Could you check a few things on this model? Use its own coordinates, in mm. Give positions to 0.01 mm unless a question says otherwise; leave off trailing zeros. Loops run counter-clockwise (first coordinate to the right, second up) from the corner with the lowest first, then second, coordinate; pieces in that order, holes last. Notation, with made-up numbers: M -30,67 L -12,67 A22 ccw -12,100 Z; hole C -17,34 d11. An arc over 180 degrees is marked long. Use a Markdown table: item, result. Add a question column.
1) Will this pin go through, and if not, where does the flat tip stop? pin 1 Ø3 at (x, y) = (0, 34.925) entering from +Z.
2) If I drill on line 1 along Y through (x, z) = (-11, 1.55) (3 decimals); line 2 along Y through (x, z) = (-8, 2.8) (3 decimals); line 3 along X through (y, z) = (30, 2.55), over which ranges is the centre line in solid material (lowest first)? Write a range as [from, to].
3) Suppose I cut it at A-A on y = 36. List the corners of the cut face in (x, z) for me (3 decimals), and give its area (3 significant figures).
```python
from build123d import *

# Parameters (mm, degrees)
F0_R     = 2.3749
F1_DEPTH = 3.175
F3_DEPTH = 25.4


with BuildPart() as f1:
    # F0 (on Top) → F1 (new body)
    with BuildSketch(Plane.XY):
        with BuildLine():
            Line((-38.1, -9.525), (38.1, -9.525))
            Line((38.1, -9.525), (38.1, 28.575))
            ThreePointArc((38.1, 28.575), (34.380256, 37.555256), (25.4, 41.275))
            Line((25.4, 41.275), (3.322108, 41.275))
            Line((3.322108, 41.275), (-25.4, 41.275))
            ThreePointArc((-25.4, 41.275), (-34.380256, 37.555256), (-38.1, 28.575))
            Line((-38.1, 28.575), (-38.1, -9.525))
        make_face()
        with Locations((0, 34.925)):
            Circle(F0_R, mode=Mode.SUBTRACT)
    extrude(amount=F1_DEPTH)

    # F2 (on face) → F3 (cut)
    with BuildSketch(Plane.XY.offset(3.175)):
        Polygon((-38.1, -7.62), (-38.1, -14.148636), (38.1, -14.148636), (38.1, -7.62), (37.1475, -9.525), (36.195, -7.62), (35.2425, -9.525), (34.29, -7.62), (33.3375, -9.525), (32.385, -7.62), (31.4325, -9.525), (30.48, -7.62), (29.5275, -9.525), (28.575, -7.62), (27.6225, -9.525), (26.67, -7.62), (25.7175, -9.525), (24.765, -7.62), (23.8125, -9.525), (22.86, -7.62), (21.9075, -9.525), (20.955, -7.62), (20.0025, -9.525), (19.05, -7.62), (18.0975, -9.525), (17.145, -7.62), (16.1925, -9.525), (15.24, -7.62), (14.2875, -9.525), (13.335, -7.62), (12.3825, -9.525), (11.43, -7.62), (10.4775, -9.525), (9.525, -7.62), (8.5725, -9.525), (7.62, -7.62), (6.6675, -9.525), (5.715, -7.62), (4.7625, -9.525), (3.81, -7.62), (2.8575, -9.525), (1.905, -7.62), (0.9525, -9.525), (0, -7.62), (-0.9525, -9.525), (-1.905, -7.62), (-2.8575, -9.525), (-3.81, -7.62), (-4.7625, -9.525), (-5.715, -7.62), (-6.6675, -9.525), (-7.62, -7.62), (-8.5725, -9.525), (-9.525, -7.62), (-10.4775, -9.525), (-11.43, -7.62), (-12.3825, -9.525), (-13.335, -7.62), (-14.2875, -9.525), (-15.24, -7.62), (-16.1925, -9.525), (-17.145, -7.62), (-18.0975, -9.525), (-19.05, -7.62), (-20.0025, -9.525), (-20.955, -7.62), (-21.9075, -9.525), (-22.86, -7.62), (-23.8125, -9.525), (-24.765, -7.62), (-25.7175, -9.525), (-26.67, -7.62), (-27.6225, -9.525), (-28.575, -7.62), (-29.5275, -9.525), (-30.48, -7.62), (-31.4325, -9.525), (-32.385, -7.62), (-33.3375, -9.525), (-34.29, -7.62), (-35.2425, -9.525), (-36.195, -7.62), (-37.1475, -9.525), align=None)
    extrude(amount=-F3_DEPTH, mode=Mode.SUBTRACT)


solid = f1.part
```
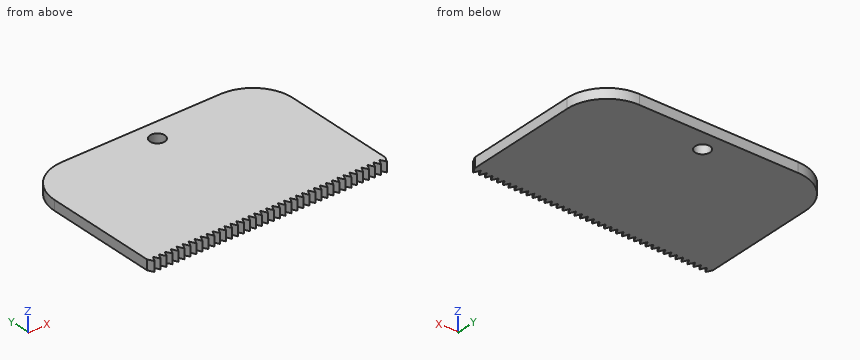
Answer block:
| question | item | result |
|---|---|---|
| 1 | pin 1 | passes through |
| 2 | line 1 | y = [-8.48, 41.275] |
| 2 | line 2 | y = [-8.38, 41.275] |
| 2 | line 3 | x = [-38.02, 38.02] |
| 3 | outline | M -35.703,0 L -2.118,0 L -2.118,3.175 L -35.703,3.175 Z; M 2.118,0 L 35.703,0 L 35.703,3.175 L 2.118,3.175 Z |
| 3 | area | 213 mm^2 |
